from build123d import *

# Parameters (mm, degrees)
SKETCH1_R           = 5.715
BOSS_EXTRUDE1_DEPTH = 25.4
SKETCH2_W           = 5.08
SKETCH2_H           = 50.8
BOSS_EXTRUDE2_DEPTH = 3.175
SKETCH3_R           = 2.159
BOSS_EXTRUDE3_DEPTH = 7.62
FILLET1_R           = 1.27
SKETCH4_W           = 3.81
SKETCH4_H           = 3.81
CUT_EXTRUDE1_DEPTH  = 7.62


with BuildPart() as part:
    # Sketch1 → Boss-Extrude1 (new body)
    with BuildSketch(Plane.XY):
        Circle(SKETCH1_R)
    extrude(amount=-BOSS_EXTRUDE1_DEPTH)

    # Sketch2 → Boss-Extrude2 (add, symmetric)
    with BuildSketch(Plane(origin=(0, 0, 0), x_dir=(0, 0, -1), z_dir=(1, 0, 0))):
        with Locations((22.86, 25.4)):
            Rectangle(SKETCH2_W, SKETCH2_H)
    extrude(amount=BOSS_EXTRUDE2_DEPTH, both=True)

    # Sketch3 → Boss-Extrude3 (add)
    with BuildSketch(Plane(origin=(0, 0, -25.4), x_dir=(-1, 0, 0), z_dir=(0, 0, -1))):
        with Locations(Location((0, 46.482, 0), (0, 0, 180))):
            Circle(SKETCH3_R)
    extrude(amount=BOSS_EXTRUDE3_DEPTH)

    # Fillet1
    fillet1_edges = [part.edges().sort_by_distance(p)[0] for p in [
        (-3.175, 27.775952441, -25.4),
        (-3.175, 50.8, -22.86),
        (0, 50.8, -25.4),
        (0, 50.8, -20.32),
        (-3.175, 27.775952441, -20.32),
        (3.175, 27.775952441, -20.32),
        (3.175, 27.775952441, -25.4),
        (3.175, 50.8, -22.86),
        (-2.159, 46.482, -33.02),
    ]]
    fillet(fillet1_edges, radius=FILLET1_R)

    # Sketch4 → Cut-Extrude1 (cut)
    with BuildSketch(Plane.XY):
        Rectangle(SKETCH4_W, SKETCH4_H)
    extrude(amount=-CUT_EXTRUDE1_DEPTH, mode=Mode.SUBTRACT)


solid = part.part
Check sheet for the modelled part. Datum: model origin and axes. Units: mm. A direction names the side the tool comes from. Round coordinates to 2 decimals unless told otherwise and drop trailing zeros. Loops run counter-clockwise (first coordinate to the right, second up) from the corner with the lowest first, then second, coordinate; pieces in that order, holes last. Notation, with made-up numbers: M -24.75,59.5 L -18.75,59.5 A24 cw -18.75,86.5 Z; hole C 38.5,-34 d9. An arc over 180 degrees is marked long. One line per question, with ' | ' between items. Start each with the question number.
Item 1: Section check A-A (y = 0). Record the boundary of the cut face in (x, z) (3 decimals).
Item 2: Scan lines: probe 1 along Z at (x, y) = (-0.5, 26); probe 2 along Y at (x, z) = (-0.5, -5.5) (3 decimals); probe 3 along Z at (x, y) = (-2.75, 3.5). Record each from-to range of solid material in increasing order.
Item 3: Release check for a two-part mould opening along X. For faces 1 (the face through (0, 0, -7.62)), 2 (the face through (-0.027, 50.438, -20.702)), 3 (the face through (-2.81, 50.42, -22.88)) record: released by +X, released by -X, zero draft, split by the parting line, or undercut.
Item 4: Section check C-C (z = -23.5). Record the boundary of the cut face in (x, y) (3 decimals).
Item 5: Gauge pin test, flat ends, axial feed: pin 1 Ø10 at (y, z) = (38, -19) entering from -X (3 decimals); pin 2 Ø1.9 at (x, y) = (-1, 1) entering from +Z; pin 3 Ø1 at (x, z) = (1, -26) entering from +Y; pin 4 Ø1.3 at (y, z) = (17.5, -23) entering from +X (3 decimals). Record the tip position at first contact, or that the pin passes through.
Item 6: Set-up check for faces 4 (the face through (2.79, 48.53, -25.04)), 5 (the face through (0, 1.905, -4)), 6 (the face through (2.79, 25.39, -25.04)), 7 (the face through (2.81, 27.45, -20.7)), 8 (the face through (0, 27, -20.32)): record each of +Z, -Z, +X, -X, +Y, -Y from which the full face is reachable in a straight line by a thin tool's end or side.
Item 7: Section check D-D (y = 34.5). Record the boundary of the cut face in (x, z) (3 decimals), and give its area (3 significant figures).
Item 8: Section check B-B (z = -3.5). Record the boundary of the cut face in (x, y) (3 decimals).
Worked out:
1) outline: M -5.715,-25.4 L 5.715,-25.4 L 5.715,0 L 1.905,0 L 1.905,-7.62 L -1.905,-7.62 L -1.905,0 L -5.715,0 Z
2) probe 1: -25.4 to -20.32 | probe 2: -5.693 to -1.905, 1.905 to 5.693 | probe 3: -25.4 to 0
3) face 1: undercut | face 2: zero draft | face 3: released by -X
4) outline: M -3.175,4.752 A5.715 ccw long 3.175,4.752 L 3.175,49.53 A1.27 ccw 1.905,50.8 L -1.905,50.8 A1.27 ccw -3.175,49.53 Z
5) pin 1: x = -3.175 | pin 2: z = 0 | pin 3: y = 48.58 | pin 4: x = 3.175
6) face 4: -Z, +X, +Y | face 5: +Z | face 6: -Z, +X | face 7: +Z, +X, +Y | face 8: +Z, +X, -X, +Y
7) outline: M -3.175,-24.13 A1.27 ccw -1.905,-25.4 L 1.905,-25.4 A1.27 ccw 3.175,-24.13 L 3.175,-21.59 A1.27 ccw 1.905,-20.32 L -1.905,-20.32 A1.27 ccw -3.175,-21.59 Z | area: 30.9 mm^2
8) outline: C 0,0 d11.43; hole M -1.905,-1.905 L 1.905,-1.905 L 1.905,1.905 L -1.905,1.905 Z
